Source: CAD feature listing. Evaluate the final solid. Frame: model axes, mm. A direction names the side the tool comes from. Round coordinates to 2 decimals unless told otherwise and drop trailing zeros. Loops run counter-clockwise (first coordinate to the right, second up) from the corner with the lowest first, then second, coordinate; pieces in that order, holes last. Notation, with made-up numbers: M 30.25,55 L 48.25,55 A23 cw 48.25,71 Z; hole C 1.25,-37.75 d10. An arc over 180 degrees is marked long. Answer as CSV lines item,"result". Start each with the question number.
```python
from build123d import *

# Parameters (mm, degrees)
F1_DEPTH = 6.35
F2_COUNT = 13
F3_R     = 2.5
F4_DEPTH = 25.4


with BuildPart() as f1:
    # F0 (on Top) → F1 (new body)
    with BuildSketch(Plane.XY):
        with BuildLine():
            ThreePointArc((7.9296197565, 23.5951858335), (6.9911317973, 23.8900761864), (6.0417249702, 24.1476546146))
            ThreePointArc((6.0417249702, 24.1476546146), (4.3226425573, 22.4330749308), (3.2648662162, 20.2476374354))
            ThreePointArc((3.2648662162, 20.2476374354), (5.7837443287, 19.6767495961), (8.2108987358, 18.7938105523))
            ThreePointArc((8.2108987358, 18.7938105523), (8.3954934616, 19.5156536929), (8.4994507341, 20.2534379554))
            ThreePointArc((8.4994507341, 20.2534379554), (8.5176465567, 20.5391701676), (8.5237154667, 20.8254168329))
            ThreePointArc((8.5237154667, 20.8254168329), (8.373521449, 22.2418004346), (7.9296197565, 23.5951858335))
        make_face()
        with BuildLine():
            ThreePointArc((4.0264902572, 14.4598933509), (-1.7431476836, 15.057566034), (-4.9211585336, 19.9100068261))
            ThreePointArc((-4.9211585336, 19.9100068261), (-12.6431262329, -16.1486077476), (20.5091729021, 0))
            ThreePointArc((20.5091729021, 0), (19.2415803806, 7.0984334598), (15.5954927821, 13.3194135761))
            ThreePointArc((15.5954927821, 13.3194135761), (9.5256046991, 10.9946956396), (4.0264902572, 14.4598933509))
        make_face()
        with BuildLine():
            ThreePointArc((3.2648662162, 20.2476374354), (-0.8451772993, 20.4917507417), (-4.9211585336, 19.9100068261))
            ThreePointArc((-4.9211585336, 19.9100068261), (-1.7431476836, 15.057566034), (4.0264902572, 14.4598933509))
            ThreePointArc((4.0264902572, 14.4598933509), (3.0384725246, 17.2738616412), (3.2648662162, 20.2476374354))
        make_face()
        with BuildLine():
            ThreePointArc((4.0264902572, 14.4598933509), (9.5256046991, 10.9946956396), (15.5954927821, 13.3194135761))
            ThreePointArc((15.5954927821, 13.3194135761), (12.2138579016, 16.4756744411), (8.2108987358, 18.7938105523))
            ThreePointArc((8.2108987358, 18.7938105523), (6.6287005247, 16.1344397874), (4.0264902572, 14.4598933509))
        make_face()
        with BuildLine():
            ThreePointArc((8.2108987358, 18.7938105523), (5.7837443287, 19.6767495961), (3.2648662162, 20.2476374354))
            ThreePointArc((3.2648662162, 20.2476374354), (3.0384725246, 17.2738616412), (4.0264902572, 14.4598933509))
            ThreePointArc((4.0264902572, 14.4598933509), (6.6287005247, 16.1344397874), (8.2108987358, 18.7938105523))
        make_face()
    extrude(amount=F1_DEPTH)

    # F2: F1 ×13 about axis
    f2_axis = Axis((0, 0, 6.35), (0, 0, 1))


with BuildPart() as f1_1:
    add(f1.part)
    for i in range(1, F2_COUNT):
        add(f1.part.rotate(f2_axis, i * 360 / F2_COUNT))

    # F3 (on face) → F4 (cut)
    with BuildSketch(Plane.XY.offset(6.35)):
        Circle(F3_R)
    extrude(amount=-F4_DEPTH, mode=Mode.SUBTRACT)


solid = f1_1.part
```
1) Mould query, pull axis X, two halves, no side actions, for faces 4 (the cylindrical face through (-18.14, -13.93, 3.13)), 5 (the cylindrical face through (-9.59, -20.77, 3.13)), 6 (the cylindrical face through (-1.08, -24.87, 3.13)), 7 (the cylindrical face through (24.556, -4.074, 3.131)). Classes: pulls with the +X half, pulls with the -X half, needs draft (parallel to the pull), parting line crosses it, or undercut.
2) Section A-A, the plane x = 1. Return loops of the section in (y, z), and give its area (3 significant figures).
3) Section B-B, the plane x = -5. Return loops of the section in (y, z).
4) Contact query for flat-ended pins moving along their axis: pin 1 Ø1.5 at (y, z) = (14.5, 4) entering from +X; pin 2 Ø2 at (y, z) = (19.5, 5) entering from +X. Output: stop coordinate, or through.
5) Section C-C, the plane y = -7. Return loops of the section in (x, z), and give its area (3 significant figures).
6) Ray query, line 1 along X through (y, z) = (18, 4.5); line 2 along X through (y, z) = (17.5, 2.25); line 3 along Y through (x, z) = (2, 5.5). Return the intervals inside material, ascending.
7) Access query for faces 1 (the cylindrical face through (22.821, -1.603, 3.131)), 2 (the cylindrical face through (-20.225, 3.403, 3.131)), 3 (the cylindrical face through (14.28, 17.87, 3.13)). Directions: +Z, -Z, +X, -X, +Y, -Y. A direction counts if a zero-diameter tool reaches every point of the face in a straight line with its end or side. Return the directions, or none.
Findings below:
1,face 4,"undercut"
1,face 5,"undercut"
1,face 6,"pulls with the -X half"
1,face 7,"pulls with the +X half"
2,outline,"M -23.21,0 L -2.29,0 L -2.29,6.35 L -23.21,6.35 Z; M 2.29,0 L 20.48,0 L 20.48,6.35 L 2.29,6.35 Z"
2,area,"248 mm²"
3,outline,"M -19.89,0 L 24.38,0 L 24.38,6.35 L -19.89,6.35 Z"
4,pin 1,"x = 17.57"
4,pin 2,"x = 16.65"
5,outline,"M -19.28,0 L 19.28,0 L 19.28,6.35 L -19.28,6.35 Z"
5,area,"245 mm²"
6,line 1,"-16.4 to -11.3, -9.83 to 9.83, 14.56 to 17.19"
6,line 2,"-16.33 to -10.86, -10.69 to 10.69, 13.63 to 17.7"
6,line 3,"-20.41 to -1.5, 1.5 to 20.41"
7,face 1,"+Z, -Z, +X"
7,face 2,"+Z, -Z, -X"
7,face 3,"+Z, -Z, +Y"
